Here's how the part is built. I have some questions about the finished solid (model axes, mm). Face numbers are marked on the shaded views. Round coordinates to 2 decimals unless told otherwise and drop trailing zeros. Write each loop counter-clockwise with the first axis right and the second up, starting at its lowest first coordinate (ties: lowest second). Pieces come first, ordered by that corner, then holes. Notation, with made-up numbers: M 3.25,14.25 L 24.25,14.25 A24 cw 24.25,42.25 Z; hole C -11.75,-9 d9. An arc over 180 degrees is marked long. Use one line per item in the form item = value. Start each with the question number.
Q1. I want a section at D-D on z = -30.5. List the corners of the cut face in (x, y) for me, and give its area (3 significant figures).
Q2. I want a section at C-C on x = 17.5. List the corners of the cut face in (y, z) for me, and give its area (3 significant figures).
Q3. I need wall thicknesses on line 1 along X through (y, z) = (5, -17.5); line 2 along Z through (x, y) = (17.5, 8.25); line 3 along Z through (x, y) = (17, 11). Which ranges of each line are inside material? Lowest first, please. Write a range as from..to.
Q4. We'd pull the mould along X, two halves only. Please class the marked faces 1, 2 and 3: +X half, -X half, draft (parallel to the pull), parting line (faces both ways), or undercut.
Q5. I want a section at A-A on z = -17.5. List the corners of the cut face in (x, y) for me.
Q6. I want a section at B-B on y = 4.5. List the corners of the cut face in (x, z) for me, and give its area (3 significant figures).
```python
from build123d import *

# Parameters (mm, degrees)
CROQUIS1_W              = 35
CROQUIS1_H              = 35
SALIENTE_EXTRUIR1_DEPTH = 18
CROQUIS2_OUTSIDE_W      = 47.534
CROQUIS2_OUTSIDE_H      = 47.534
CORTAR_EXTRUIR2_DEPTH   = 18
CROQUIS3_R              = 2.5
CORTAR_EXTRUIR3_DEPTH   = 19


with BuildPart() as part:
    # Croquis1 → Saliente-Extruir1 (new body)
    with BuildSketch(Plane(origin=(0, 0, 0), x_dir=(1, 0, 0), z_dir=(0, 1, 0))):
        with Locations((17.5, 17.5)):
            Rectangle(CROQUIS1_W, CROQUIS1_H)
    extrude(amount=SALIENTE_EXTRUIR1_DEPTH)

    # Croquis2 outside → Cortar-Extruir2 (cut)
    with BuildSketch(Plane(origin=(0, 18, 0), x_dir=(1, 0, 0), z_dir=(0, 1, 0))):
        with Locations((17.5, 17.5)):
            Rectangle(CROQUIS2_OUTSIDE_W, CROQUIS2_OUTSIDE_H)
        Polygon((5.30151519, 35), (0, 29.69848481), (0, 5.30151519), (5.30151519, 0), (29.69848481, 0), (35, 5.30151519), (35, 29.69848481), (29.69848481, 35), align=None, mode=Mode.SUBTRACT)
    extrude(amount=-CORTAR_EXTRUIR2_DEPTH, mode=Mode.SUBTRACT)

    # Croquis3 → Cortar-Extruir3 (cut, through all)
    with BuildSketch(Plane(origin=(0, 18, 0), x_dir=(1, 0, 0), z_dir=(0, 1, 0))):
        with Locations((17.5, 17.5)):
            Circle(CROQUIS3_R)
    extrude(amount=-CORTAR_EXTRUIR3_DEPTH, mode=Mode.SUBTRACT)


solid = part.part
```
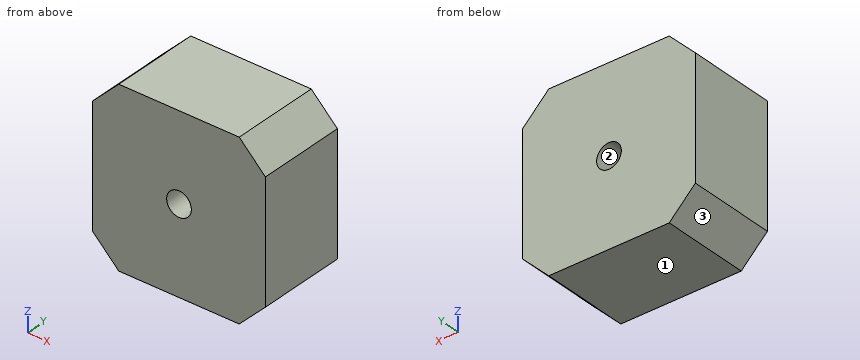
Reported:
q1.outline = M 0.8,0 L 34.2,0 L 34.2,18 L 0.8,18 Z
q1.area = 601 mm^2
q2.outline = M 0,-35 L 18,-35 L 18,-20 L 0,-20 Z; M 0,-15 L 18,-15 L 18,0 L 0,0 Z
q2.area = 540 mm^2
q3.line_1 = 0..15, 20..35
q3.line_2 = -35..-20, -15..0
q3.line_3 = -35..-19.95, -15.05..0
q4.face_1 = draft
q4.face_2 = undercut
q4.face_3 = -X half
q5.outline = M 0,0 L 15,0 L 15,18 L 0,18 Z; M 20,0 L 35,0 L 35,18 L 20,18 Z
q6.outline = M 0,-29.7 L 5.3,-35 L 29.7,-35 L 35,-29.7 L 35,-5.3 L 29.7,0 L 5.3,0 L 0,-5.3 Z; hole C 17.5,-17.5 d5
q6.area = 1,150 mm^2
